from build123d import *

# Parameters (mm, degrees)
SKETCH2_R           = 1
SKETCH2_R_2         = 13
SKETCH2_R_3         = 11.5
BOSS_EXTRUDE1_DEPTH = 1.6
CHAMFER1_SIZE       = 10


with BuildPart() as part:
    # Sketch2 → Boss-Extrude1 (new body)
    with BuildSketch(Plane(origin=(0, 0, 0), x_dir=(1, 0, 0), z_dir=(0, 1, 0))):
        Polygon((0, 21.5), (51.666666667, 21.5), (51.666666667, 18.5), (91.666666667, 18.5), (91.666666667, 21.5), (125, 21.5), (125, -21.5), (91.666666667, -21.5), (91.666666667, -18.5), (51.666666667, -18.5), (51.666666667, -21.5), (0, -21.5), align=None)
        with Locations((19.37, 13)):
            Circle(SKETCH2_R, mode=Mode.SUBTRACT)
        with Locations((87.87, 13)):
            Circle(SKETCH2_R, mode=Mode.SUBTRACT)
        with Locations((87.87, -13)):
            Circle(SKETCH2_R, mode=Mode.SUBTRACT)
        with Locations((19.37, -13)):
            Circle(SKETCH2_R, mode=Mode.SUBTRACT)
        with Locations((39.37, 0)):
            Circle(SKETCH2_R_2, mode=Mode.SUBTRACT)
        with Locations((107.87, 0)):
            Circle(SKETCH2_R_2, mode=Mode.SUBTRACT)
        with Locations((71.666666667, 0)):
            Circle(SKETCH2_R_3, mode=Mode.SUBTRACT)
    extrude(amount=BOSS_EXTRUDE1_DEPTH)

    # Chamfer1
    chamfer1_edges = [part.edges().sort_by_distance(p)[0] for p in [
        (0, 0.8, 21.5),
        (0, 0.8, -21.5),
        (125, 0.8, -21.5),
        (125, 0.8, 21.5),
    ]]
    chamfer(chamfer1_edges, length=CHAMFER1_SIZE)


solid = part.part
Can you work these out from the model? Positions are in its coordinate system, mm. Coordinates: 2 decimals unless noted, no trailing zeros. Order: outer loops, then holes, each group sorted by start corner. A loop starts at its lowest first (then second) coordinate and runs counter-clockwise, first axis right, second up. Notation, with made-up numbers: (-4, 62.5) - (2, 62.5) arc R33 cw to (2, 95.5) - close; hole circle Ø2 at (29, -11.75). An arc over 180 degrees is marked (long way). Answer as a JSON object with one key per item and string values. Group by question number.
Q1. Will these pins go through, and if not, where does the flat tip stop? P1, Ø0.5, axis at y = 1, z = 20, coming from the +X side; P2, Ø10, axis at x = 33.5, z = -6.5, coming from the -Y side; P3, Ø1.2, axis at x = 87.87, z = 13, coming from the -Y side; P4, Ø0.5, axis at y = 1, z = 20.5, coming from the -X side.
Q2. I need wall thicknesses on line 1 (Z direction, x = 39.37, y = 1); line 2 (X direction, y = 1.5, z = -10); line 3 (X direction, y = 0.6, z = 2). Which ranges of each line are inside material? Lowest first, please. Write a range as from..to.
Q3. Imagine slicing it at A-A (x = 107.87). Please give me the cut outline in (y, z), and give its area (3 significant figures).
Q4. Imagine slicing it at B-B (y = 0.25). Please give me the cut outline in (x, z).
Q5. We'd pull the mould along X, two halves only. Please class faces 1 (the face through (5.1, 0.8, 16.6)), 2 (the face through (26.383, 0.789, -0.572)), 3 (the face through (49, 1.6, 9)), 4 (the face through (120.1, 0.8, -16.4)): +X half, -X half, draft (parallel to the pull), parting line (faces both ways), or undercut.
Q6. Imagine slicing it at C-C (z = 6.5). Please give me the cut outline in (x, y).
Q7. Imagine slicing it at D-D (z = -3). Please give me the cut outline in (x, y).
Determined:
{
 "1": {"P1": "stops at x = 116.75", "P2": "stops at y = 0", "P3": "passes through", "P4": "stops at x = 8.75"},
 "2": {"line 1": "z = -21.5..-13, 13..21.5", "line 2": "x = 0..31.06, 47.68..65.99, 77.35..99.56, 116.18..125", "line 3": "x = 0..26.52, 52.22..60.34, 82.99..95.02, 120.72..125"},
 "3": {"outline": "(0, -21.5) - (1.6, -21.5) - (1.6, -13) - (0, -13) - close; (0, 13) - (1.6, 13) - (1.6, 21.5) - (0, 21.5) - close", "area": "27.2 mm2"},
 "4": {"outline": "(0, -11.5) - (10, -21.5) - (51.67, -21.5) - (51.67, -18.5) - (91.67, -18.5) - (91.67, -21.5) - (115, -21.5) - (125, -11.5) - (125, 11.5) - (115, 21.5) - (91.67, 21.5) - (91.67, 18.5) - (51.67, 18.5) - (51.67, 21.5) - (10, 21.5) - (0, 11.5) - close; hole circle Ø2 at (19.37, -13); hole circle Ø2 at (19.37, 13); hole circle Ø26 at (39.37, 0); hole circle Ø23 at (71.67, 0); hole circle Ø2 at (87.87, -13); hole circle Ø2 at (87.87, 13); hole circle Ø26 at (107.87, 0)"},
 "5": {"face 1": "-X half", "face 2": "undercut", "face 3": "draft", "face 4": "+X half"},
 "6": {"outline": "(0, 0) - (28.11, 0) - (28.11, 1.6) - (0, 1.6) - close; (50.63, 0) - (62.18, 0) - (62.18, 1.6) - (50.63, 1.6) - close; (81.15, 0) - (96.61, 0) - (96.61, 1.6) - (81.15, 1.6) - close; (119.13, 0) - (125, 0) - (125, 1.6) - (119.13, 1.6) - close"},
 "7": {"outline": "(0, 0) - (26.72, 0) - (26.72, 1.6) - (0, 1.6) - close; (52.02, 0) - (60.56, 0) - (60.56, 1.6) - (52.02, 1.6) - close; (82.77, 0) - (95.22, 0) - (95.22, 1.6) - (82.77, 1.6) - close; (120.52, 0) - (125, 0) - (125, 1.6) - (120.52, 1.6) - close"}
}
